Build history of the part. All positions in model axes, mm. A direction names the side the tool comes from. Round coordinates to 2 decimals unless told otherwise and drop trailing zeros. Write each loop counter-clockwise with the first axis right and the second up, starting at its lowest first coordinate (ties: lowest second). Pieces come first, ordered by that corner, then holes.
Item 1: 3-axis set-ups, long thin cutter, end or side, ignore diameter. For faces 4 (the flat face through (5.092, -10, 8)), 5 (the flat face through (-1, -2, 8)), 6 (the flat face through (0, -17, 6.651)): which of +Z, -Z, +X, -X, +Y, -Y reach the whole face in a straight line?
Item 2: Drop flat-ended pins along their axis: pin 1 Ø1 at (x, z) = (0, 2) entering from +Y; pin 2 Ø1 at (x, z) = (0, 8) entering from +Y; pin 3 Ø3 at (x, y) = (-0.5, -20.5) entering from -Z. Give the stop position or say it passes through.
Item 3: Wall check: probe 1 along Z at (x, y) = (2.75, -13.5); probe 2 along X at (y, z) = (-38.5, 6.5); probe 3 along Y at (x, z) = (0, 3.5). Give the ranges that are in metal, low to high.
Item 4: Band-saw the part on A-A, the plane z = 8.25. Write the cut outline in (x, y).
Item 5: Band-saw the part on C-C, the plane x = 3. Write the cut outline in (y, z).
Item 6: Mould opens along Y. For faces 1 (the flat face through (0.02, -37.86, 0.7)), 2 (the flat face through (3, 0, 8)), 3 (the flat face through (-2.5, -33.22, 7.15)) say: +Y half, -Y half, draft (parallel to the pull), parting line (faces both ways), or undercut.
Item 7: Band-saw the part on B-B, the plane y = -16. Write the cut outline in (x, z).
```python
from build123d import *

# Parameters (mm, degrees)
F1_DEPTH = 10
F3_DEPTH = 12.5
F5_DEPTH = 12.5
F7_DEPTH = 74


with BuildPart() as f1:
    # F0 (on Top) → F1 (new body)
    with BuildSketch(Plane.XY):
        Polygon((0, -41.570846), (0, 0), (-5.092436, 0), (-5.092436, -20.467674), (-0.80141, -41.570846), align=None)
        Polygon((5.092436, 0), (0, 0), (0, -41.570846), (0.80141, -41.570846), (5.092436, -20.467674), align=None)
    extrude(amount=F1_DEPTH)

    # F2 (on Right) → F3 (cut, symmetric)
    with BuildSketch(Plane.YZ):
        Polygon((-37.5918, -12.62699), (0, -8.964199), (0, 6.650857), (-33.736233, 6.650857), (-37.5918, 0), align=None)
    extrude(amount=F3_DEPTH, both=True, mode=Mode.SUBTRACT)

    # F4 (on Right) → F5 (cut, symmetric)
    with BuildSketch(Plane.YZ):
        Polygon((-40.562909, 1.382743), (-41.8077, -0.256735), (-43.113209, -1.562245), (-35.917722, -1.926574), (-37.648283, 0), (-38.073331, 1.413104), (-38.771629, 0), (-39.196678, 1.322022), (-40.1075, 0), align=None)
    extrude(amount=F5_DEPTH, both=True, mode=Mode.SUBTRACT)

    # F6 (on Top) → F7 (cut)
    with BuildSketch(Plane.XY):
        Polygon((1, 4.449242), (0, 4.449242), (0, -4.97661), (1, -4.97661), (1, 0), align=None)
        Polygon((0, -4.97661), (0, 4.449242), (-1, 4.449242), (-1, 0), (-1, -4.97661), align=None)
    extrude(amount=F7_DEPTH, mode=Mode.SUBTRACT)


solid = f1.part
```
Results:
1. face 4: +Z, -Z, +X, +Y, -Y
1. face 5: +Z, -Z, +Y
1. face 6: -Z, +X, -X, +Y
2. pin 1: stops at y = -36.14
2. pin 2: stops at y = -4.98
2. pin 3: stops at z = 6.65
3. probe 1: z = 6.65 to 10
3. probe 2: x = -1.43 to 1.43
3. probe 3: y = -41.57 to -35.56
4. outline: (-5.09, -20.47) - (-0.8, -41.57) - (0.8, -41.57) - (5.09, -20.47) - (5.09, 0) - (1, 0) - (1, -4.98) - (-1, -4.98) - (-1, 0) - (-5.09, 0) - close
5. outline: (-30.76, 6.65) - (0, 6.65) - (0, 10) - (-30.76, 10) - close
6. face 1: undercut
6. face 2: +Y half
6. face 3: -Y half
7. outline: (-5.09, 6.65) - (5.09, 6.65) - (5.09, 10) - (-5.09, 10) - close
